```python
from build123d import *

# Parameters (mm, degrees)
SKETCH1_R      = 5.5
EXTRUDE1_DEPTH = 73
EXTRUDE2_DEPTH = 8
SKETCH3_R      = 14.116748978
SKETCH3_R_2    = 7
EXTRUDE3_DEPTH = 0.5
SKETCH4_R      = 19.693652211
SKETCH4_R_2    = 4.5
EXTRUDE4_DEPTH = 5
CHAMFER1_SIZE  = 1
SKETCH5_R      = 25.58893004
SKETCH5_R_2    = 8
EXTRUDE5_DEPTH = 1
CHAMFER2_SIZE  = 1


# Some blends are built 0.0001 mm under size
with BuildPart() as part:
    # Sketch1 → Extrude1 (new body)
    with BuildSketch(Plane(origin=(0, 0, 0), x_dir=(1, 0, 0), z_dir=(0, 1, 0))):
        with Locations(Location((0, 0, 0), (0, 0, 270))):
            Circle(SKETCH1_R)
    extrude(amount=EXTRUDE1_DEPTH)

    # Sketch2 → Extrude2 (add)
    with BuildSketch(Plane(origin=(0, 73, 0), x_dir=(1, 0, 0), z_dir=(0, 1, 0))):
        Polygon((8, -4.618802154), (8, 4.618802154), (0, 9.237604307), (-8, 4.618802154), (-8, -4.618802154), (0, -9.237604307), align=None)
    extrude(amount=EXTRUDE2_DEPTH)

    # Sketch3 → Extrude3 (cut)
    with BuildSketch(Plane.XZ.offset(-73)):
        Circle(SKETCH3_R)
        with Locations(Location((0, 0, 0), (0, 0, 270))):
            Circle(SKETCH3_R_2, mode=Mode.SUBTRACT)
    extrude(amount=-EXTRUDE3_DEPTH, mode=Mode.SUBTRACT)

    # Sketch4 → Extrude4 (cut)
    with BuildSketch(Plane.XZ):
        Circle(SKETCH4_R)
        with Locations(Location((0, 0, 0), (0, 0, 270))):
            Circle(SKETCH4_R_2, mode=Mode.SUBTRACT)
    extrude(amount=-EXTRUDE4_DEPTH, mode=Mode.SUBTRACT)

    # Chamfer1
    chamfer1_edges = [part.edges().sort_by_distance(p)[0] for p in [
        (0, 5, -5.5),
    ]]
    chamfer(chamfer1_edges, length=CHAMFER1_SIZE - 0.0001)  # a hair under: the kernel refuses the full size

    # Sketch5 → Extrude5 (cut)
    with BuildSketch(Plane(origin=(0, 81, 0), x_dir=(1, 0, 0), z_dir=(0, 1, 0))):
        Circle(SKETCH5_R)
        with Locations(Location((0, 0, 0), (0, 0, 270))):
            Circle(SKETCH5_R_2, mode=Mode.SUBTRACT)
    extrude(amount=-EXTRUDE5_DEPTH, mode=Mode.SUBTRACT)

    # Chamfer2
    # the kernel refuses this chamfer: 1 mm, written as the material it adds along each edge
    with BuildSketch(Plane(origin=(0, 80, 0), x_dir=(0.5000000000000043, 0, -0.8660254037844362), z_dir=(0.8660254037844362, 0, 0.5000000000000043))) as chamfer2_piece_1_section:
        Polygon((8, CHAMFER2_SIZE), (8 + CHAMFER2_SIZE, 0), (8, 0), align=None)
    chamfer2_piece_1 = revolve(axis=Axis((0, 80, 0), (0, 1, 0)), revolution_arc=60, mode=Mode.PRIVATE)
    chamfer2_piece_1 = split(chamfer2_piece_1, bisect_by=Plane(origin=(-0.488712857, 80.376891688, -8.955445807), z_dir=(0.49999999999999606, 0, 0.8660254037844412)), keep=Keep.TOP, mode=Mode.PRIVATE)
    chamfer2_piece_1 = split(chamfer2_piece_1, bisect_by=Plane(origin=(0.488712857, 80.376891688, -8.955445807), z_dir=(-0.500000000000004, 0, 0.8660254037844364)), keep=Keep.TOP, mode=Mode.PRIVATE)
    add(chamfer2_piece_1)
    with BuildSketch(Plane(origin=(0, 80, 0), x_dir=(-0.4999999999999957, 0, -0.8660254037844412), z_dir=(0.8660254037844412, 0, -0.4999999999999957))) as chamfer2_piece_2_section:
        Polygon((8, CHAMFER2_SIZE), (8 + CHAMFER2_SIZE, 0), (8, 0), align=None)
    chamfer2_piece_2 = revolve(axis=Axis((0, 80, 0), (0, 1, 0)), revolution_arc=60, mode=Mode.PRIVATE)
    chamfer2_piece_2 = split(chamfer2_piece_2, bisect_by=Plane(origin=(-8, 80.376891688, -4.054485154), z_dir=(1, 0, 0)), keep=Keep.TOP, mode=Mode.PRIVATE)
    chamfer2_piece_2 = split(chamfer2_piece_2, bisect_by=Plane(origin=(-7.511287143, 80.376891688, -4.900960653), z_dir=(0.49999999999999606, 0, 0.8660254037844412)), keep=Keep.TOP, mode=Mode.PRIVATE)
    add(chamfer2_piece_2)
    with BuildSketch(Plane(origin=(0, 80, 0), x_dir=(-1, 0, 0), z_dir=(0, 0, -1))) as chamfer2_piece_3_section:
        Polygon((8, CHAMFER2_SIZE), (8 + CHAMFER2_SIZE, 0), (8, 0), align=None)
    chamfer2_piece_3 = revolve(axis=Axis((0, 80, 0), (0, 1, 0)), revolution_arc=60, mode=Mode.PRIVATE)
    chamfer2_piece_3 = split(chamfer2_piece_3, bisect_by=Plane(origin=(-7.511287143, 80.376891688, 4.900960653), z_dir=(0.5000000000000039, 0, -0.8660254037844365)), keep=Keep.TOP, mode=Mode.PRIVATE)
    chamfer2_piece_3 = split(chamfer2_piece_3, bisect_by=Plane(origin=(-8, 80.376891688, 4.054485154), z_dir=(1, 0, 0)), keep=Keep.TOP, mode=Mode.PRIVATE)
    add(chamfer2_piece_3)
    with BuildSketch(Plane(origin=(0, 80, 0), x_dir=(1, 0, 0), z_dir=(0, 0, 1))) as chamfer2_piece_4_section:
        Polygon((8, CHAMFER2_SIZE), (8 + CHAMFER2_SIZE, 0), (8, 0), align=None)
    chamfer2_piece_4 = revolve(axis=Axis((0, 80, 0), (0, 1, 0)), revolution_arc=60, mode=Mode.PRIVATE)
    chamfer2_piece_4 = split(chamfer2_piece_4, bisect_by=Plane(origin=(8, 80.376891688, -4.054485154), z_dir=(-1, 0, 0)), keep=Keep.TOP, mode=Mode.PRIVATE)
    chamfer2_piece_4 = split(chamfer2_piece_4, bisect_by=Plane(origin=(7.511287143, 80.376891688, -4.900960653), z_dir=(-0.500000000000004, 0, 0.8660254037844364)), keep=Keep.TOP, mode=Mode.PRIVATE)
    add(chamfer2_piece_4)
    with BuildSketch(Plane(origin=(0, 80, 0), x_dir=(-0.5000000000000046, 0, 0.8660254037844362), z_dir=(-0.8660254037844362, 0, -0.5000000000000046))) as chamfer2_piece_5_section:
        Polygon((8, CHAMFER2_SIZE), (8 + CHAMFER2_SIZE, 0), (8, 0), align=None)
    chamfer2_piece_5 = revolve(axis=Axis((0, 80, 0), (0, 1, 0)), revolution_arc=30, mode=Mode.PRIVATE)
    chamfer2_piece_5 = split(chamfer2_piece_5, bisect_by=Plane(origin=(-1.40811023, 80.376891688, 8.424631487), z_dir=(0.5000000000000039, 0, -0.8660254037844365)), keep=Keep.TOP, mode=Mode.PRIVATE)
    add(chamfer2_piece_5)
    with BuildSketch(Plane(origin=(0, 80, 0), x_dir=(0.4999999999999962, 0, 0.8660254037844408), z_dir=(-0.8660254037844408, 0, 0.4999999999999962))) as chamfer2_piece_6_section:
        Polygon((8 + CHAMFER2_SIZE, 0), (8, CHAMFER2_SIZE), (8, 0), align=None)
    chamfer2_piece_6 = revolve(axis=Axis((0, 80, 0), (0, 1, 0)), revolution_arc=60, mode=Mode.PRIVATE)
    chamfer2_piece_6 = split(chamfer2_piece_6, bisect_by=Plane(origin=(8, 80.376891688, 4.054485154), z_dir=(-1, 0, 0)), keep=Keep.TOP, mode=Mode.PRIVATE)
    chamfer2_piece_6 = split(chamfer2_piece_6, bisect_by=Plane(origin=(7.511287143, 80.376891688, 4.900960653), z_dir=(-0.4999999999999963, 0, -0.866025403784441)), keep=Keep.TOP, mode=Mode.PRIVATE)
    add(chamfer2_piece_6)
    with BuildSketch(Plane(origin=(0, 80, 0), x_dir=(0, 0, 1), z_dir=(-1, 0, 0))) as chamfer2_piece_7_section:
        Polygon((8, CHAMFER2_SIZE), (8 + CHAMFER2_SIZE, 0), (8, 0), align=None)
    chamfer2_piece_7 = revolve(axis=Axis((0, 80, 0), (0, 1, 0)), revolution_arc=30, mode=Mode.PRIVATE)
    chamfer2_piece_7 = split(chamfer2_piece_7, bisect_by=Plane(origin=(1.40811023, 80.376891688, 8.424631487), z_dir=(-0.4999999999999963, 0, -0.866025403784441)), keep=Keep.TOP, mode=Mode.PRIVATE)
    add(chamfer2_piece_7)


solid = part.part
```
Work out the finished part from the listing and answer in its coordinate system (mm). A direction names the side the tool comes from. Give positions to 0.01 mm unless a question says otherwise; leave off trailing zeros. Loops run counter-clockwise (first coordinate to the right, second up) from the corner with the lowest first, then second, coordinate; pieces in that order, holes last. Notation, with made-up numbers: (31.5, 7) -> (83.5, 7) arc R11 cw to (83.5, 26) -> close; hole circle Ø5 at (-5, 5.25). An arc over 180 degrees is marked (long way). Use CSV: the item, a comma, the result in double quotes.
1. The part is cut by section A-A (y = 16). Write down the section's boundary in (x, z), then the cut area to 3 significant figures.
Found:
outline,"circle Ø11 at (0, 0)"
area,"95.0 mm^2"
2. A tool of negligible diameter and unlimited length cuts with its end or side. For faces 1 (the flat face through (0, 81, 0)), 2 (the flat face through (-4, 73, 4)), from which of +Z, -Z, +X, -X, +Y, -Y can it reach the whole face along a straight path? Write none if from no direction.
Found:
face 1,"+Z, -Z, +X, -X, +Y"
face 2,"-Y"
3. Straight lines are drawn through the part: line 1 (Y direction, x = -5.5, z = -4.75); line 2 (Y direction, x = 5.25, z = -2.25); line 3 (Z direction, x = 4, y = 64). For each, find the intervals that lie inside material, in ascending order.
Found:
line 1,"73.5 to 81"
line 2,"73 to 81"
line 3,"-3.77 to 3.77"
4. Flat-ended cylindrical pins translate along their axes: pin 1 Ø10 at (y, z) = (12, -1.5) entering from -X; pin 2 Ø1.5 at (x, y) = (2.5, 51) entering from +Z; pin 3 Ø5 at (y, z) = (53.5, 4.5) entering from +X; pin 4 Ø2 at (x, z) = (3.5, 3) entering from -Y. Find the tip coordinate at first contact, or state that the pin passes through.
Found:
pin 1,"x = -5.5"
pin 2,"z = 5.21"
pin 3,"x = 5.12"
pin 4,"y = 0"
